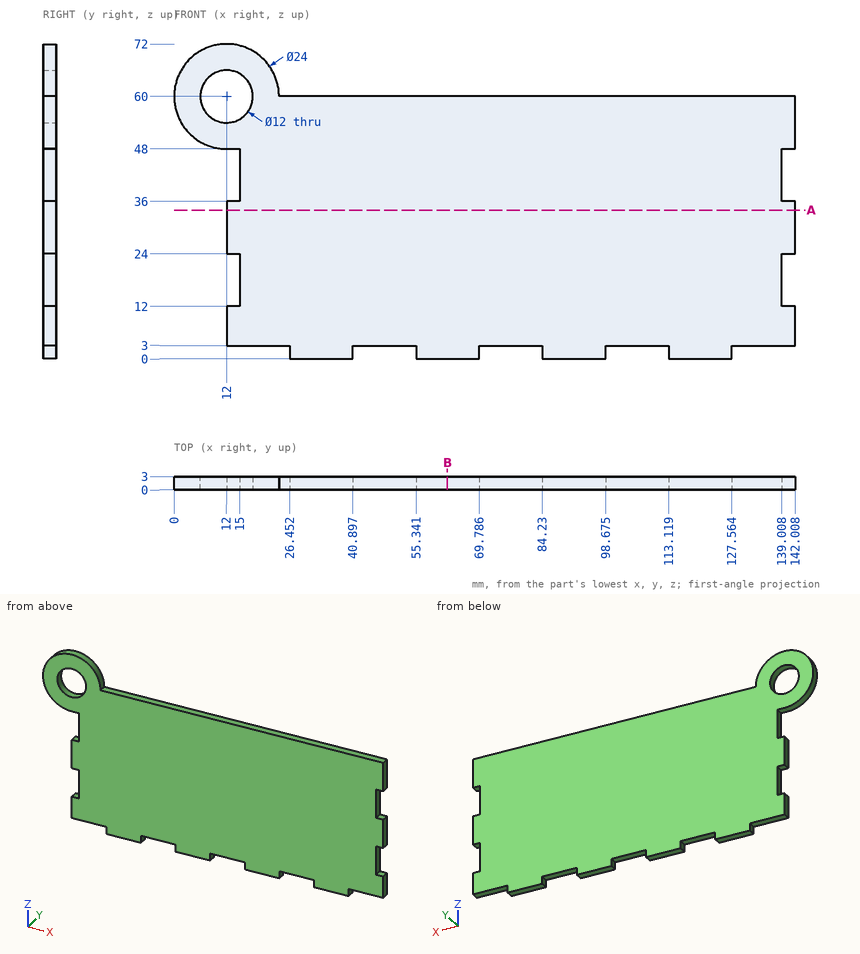
Geometry: see drawing. Coordinates: mm, zero at the bounding-box minimum. Round coordinates to 2 decimals unless told otherwise and drop trailing zeros. Loops run counter-clockwise (first coordinate to the right, second up) from the corner with the lowest first, then second, coordinate; pieces in that order, holes last.
(1) Contact query for flat-ended pins moving along their axis: pin 1 Ø1.5 at (x, y) = (140, 1.5) entering from -Z; pin 2 Ø1.5 at (y, z) = (1, 32.5) entering from -X; pin 3 Ø1.5 at (y, z) = (1, 41.5) entering from +X. Output: stop coordinate, or through.
From the geometry:
pin 1: stops at z = 3
pin 2: stops at x = 12
pin 3: stops at x = 139.01
(2) Section query A-A (z = 34). Output: boundary loops of the cut face in (x, y).
From the geometry:
outline: (12, 0) - (142.01, 0) - (142.01, 3) - (12, 3) - close
(3) Section query B-B (x = 62.5). Output: boundary loops of the cut face in (y, z), and give its area (3 significant figures).
From the geometry:
outline: (0, 0) - (3, 0) - (3, 60) - (0, 60) - close
area: 180 mm2
(4) Material intervals for probe 1 along X at (y, z) = (2.55, 47); probe 2 along Z at (x, y) = (42, 2.55); probe 3 along Z at (x, y) = (57, 2.4), sorted ascending.
From the geometry:
probe 1: x = 15 to 139.01
probe 2: z = 3 to 60
probe 3: z = 0 to 60
